The figure shows three views and two pictorial views of one solid part (mm, origin at its lowest corner). Answer the questions. A direction names the side the tool comes from. Round coordinates to 2 decimals unless told otherwise and drop trailing zeros. Order: outer loops, then holes, each group sorted by start corner. A loop starts at its lowest first (then second) coordinate and runs counter-clockwise, first axis right, second up. Notation, with made-up numbers: (-8.5, 84) - (37.5, 84) arc R30 ccw to (37.5, 117) - close; hole circle Ø5 at (-26.75, 7). An arc over 180 degrees is marked (long way). Write item = value, one per line.
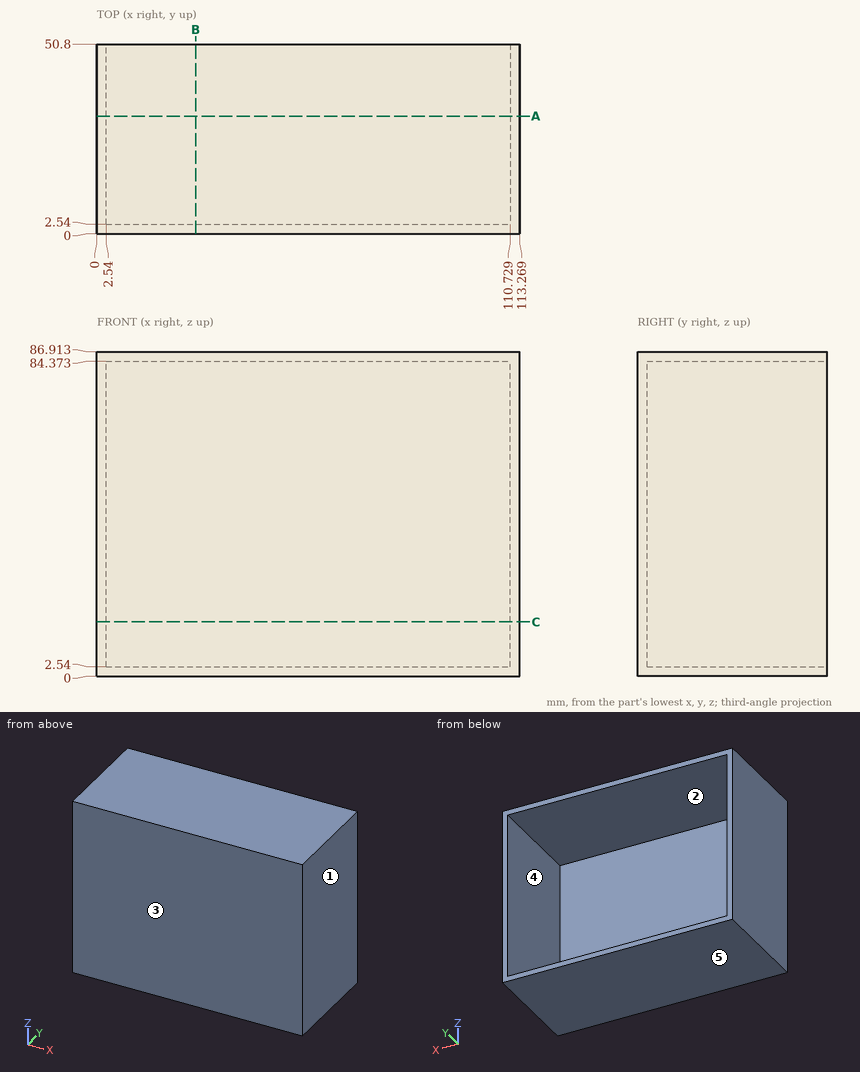
Q1. Find the intervals of material crossed by line 1 (Z direction, x = 42.5, y = 34.5); line 2 (X direction, y = 23.5, z = 80); line 3 (Y direction, x = 67, z = 77), in increasing order. Write a range as from..to.
Model answer:
line_1 = 0..2.54, 84.37..86.91
line_2 = 0..2.54, 110.73..113.27
line_3 = 0..2.54
Q2. A flat-ended cylindrical pin translates along its axis: P1, Ø2, axis at x = 38.5, z = 60, coming from the +Y side. Find the tip coordinate at first contact, or state that the pin passes through.
Model answer:
P1 = 2.54
Q3. Determine the mould class of the marked faces 3, 4 and 5 for opening direction Z: released by +Z, released by -Z, zero draft, split by the parting line, or undercut.
Model answer:
face_3 = zero draft
face_4 = undercut
face_5 = released by -Z
Q4. For the marked faces 1 and 2, determine the directions among +Z, -Z, +X, -X, +Y, -Y from which every point of the face is accessible in a straight line to the end or side of a thin tool.
Model answer:
face_1 = +Z, -Z, +X, +Y, -Y
face_2 = +Y
Q5. Section A-A on y = 31.5 is taken. Determine the outline of the cut face in (x, z), then the cut area to 3 significant figures.
Model answer:
outline = (0, 0) - (113.27, 0) - (113.27, 86.91) - (0, 86.91) - close; hole (2.54, 2.54) - (110.73, 2.54) - (110.73, 84.37) - (2.54, 84.37) - close
area = 991 mm^2
Q6. Section B-B on x = 26.5 is taken. Determine the outline of the cut face in (y, z).
Model answer:
outline = (0, 0) - (50.8, 0) - (50.8, 2.54) - (2.54, 2.54) - (2.54, 84.37) - (50.8, 84.37) - (50.8, 86.91) - (0, 86.91) - close
Q7. Section C-C on z = 14.5 is taken. Determine the outline of the cut face in (x, y), then the cut area to 3 significant figures.
Model answer:
outline = (0, 0) - (113.27, 0) - (113.27, 50.8) - (110.73, 50.8) - (110.73, 2.54) - (2.54, 2.54) - (2.54, 50.8) - (0, 50.8) - close
area = 533 mm^2
